from build123d import *

# Parameters (mm, degrees)
F0_W     = 500
F0_H     = 300
F1_DEPTH = 31.75
F2_R     = 1.5
F3_DEPTH = 31.751
F5_DEPTH = 12
F8_DEPTH = 31.751
F9_DEPTH = 19.05


# Not quite as in the source:
# - a length typed as a fraction of an inch, garbled in the dataset ("3 / 203.2 mm" for 3/8 in), is restored


with BuildPart() as f1:
    # F0 (on Top) → F1 (new body)
    with BuildSketch(Plane.XY):
        Rectangle(F0_W, F0_H)
    extrude(amount=-F1_DEPTH)

    # F2 (on Top) → F3 (cut, through all)
    with BuildSketch(Plane.XY):
        with Locations((-214.6335691214, 119.7834908962)):
            Circle(F2_R)
        with Locations((-214.6335691214, -117.7065091038)):
            Circle(F2_R)
        with Locations((207.7684308786, 119.7834908962)):
            Circle(F2_R)
        with Locations((207.7684308786, -117.7065091038)):
            Circle(F2_R)
        with Locations((630.1704308786, 119.7834908962)):
            Circle(F2_R)
        with Locations((630.1704308786, -117.7065091038)):
            Circle(F2_R)
    extrude(amount=-F3_DEPTH, mode=Mode.SUBTRACT)

    # F4 (on Top) → F5 (cut)
    with BuildSketch(Plane.XY):
        with BuildLine():
            ThreePointArc((-193.759300375, -80.4257169581), (-188.1796845566, -93.8961011397), (-174.709300375, -99.4757169581))
            Line((-174.709300375, -99.4757169581), (161.840699625, -99.4757169581))
            ThreePointArc((161.840699625, -99.4757169581), (175.3110838066, -93.8961011397), (180.890699625, -80.4257169581))
            Line((180.890699625, -80.4257169581), (180.890699625, 62.4492830419))
            ThreePointArc((180.890699625, 62.4492830419), (175.3110838066, 75.9196672235), (161.840699625, 81.4992830419))
            Line((161.840699625, 81.4992830419), (-174.709300375, 81.4992830419))
            ThreePointArc((-174.709300375, 81.4992830419), (-188.1796845566, 75.9196672235), (-193.759300375, 62.4492830419))
            Line((-193.759300375, 62.4492830419), (-193.759300375, -80.4257169581))
        make_face()
        with BuildLine():
            Line((210.890699625, 104.8424765468), (190.890699625, 104.8424765468))
            Line((190.890699625, 104.8424765468), (190.890699625, 11.4992830419))
            ThreePointArc((190.890699625, 11.4992830419), (200.890699625, 1.4992830419), (210.890699625, 11.4992830419))
            Line((210.890699625, 11.4992830419), (210.890699625, 104.8424765468))
        make_face()
    extrude(amount=-F5_DEPTH, mode=Mode.SUBTRACT)

    # F7 (on face) → F8 (cut, through all)
    with BuildSketch(Plane.XY):
        with BuildLine():
            Line((-174.709300375, -93.1257169581), (140.1676505526, -93.1257169581))
            Line((140.1676505526, -93.1257169581), (163.0281784434, -99.438670281))
            ThreePointArc((163.0281784434, -99.438670281), (175.7245746513, -93.4695091312), (180.890699625, -80.4257169581))
            Line((180.890699625, -80.4257169581), (180.890699625, 56.0992830419))
            Line((180.890699625, 56.0992830419), (154.220699625, 81.4992830419))
            Line((154.220699625, 81.4992830419), (-168.359300375, 81.4992830419))
            Line((-168.359300375, 81.4992830419), (-187.409300375, 62.4492830419))
            Line((-187.409300375, 62.4492830419), (-193.759300375, 56.0992830419))
            Line((-193.759300375, 56.0992830419), (-193.759300375, -74.0757169581))
            Line((-193.759300375, -74.0757169581), (-174.709300375, -93.1257169581))
        make_face()
    extrude(amount=-F8_DEPTH, mode=Mode.SUBTRACT)

    # F6 (on Top) → F9 (cut)
    with BuildSketch(Plane.XY):
        with BuildLine():
            ThreePointArc((-161.120300375, 111.4992830419), (-166.7055905698, 109.0628082362), (-168.7191172889, 103.3114965432))
            Line((-168.7191172889, 103.3114965432), (-167.089300375, 81.4992830419))
            Line((-167.089300375, 81.4992830419), (-93.429300375, 81.4992830419))
            Line((-93.429300375, 81.4992830419), (-91.799483461, 103.3114965432))
            ThreePointArc((-91.799483461, 103.3114965432), (-93.8130101802, 109.0628082362), (-99.398300375, 111.4992830419))
            Line((-99.398300375, 111.4992830419), (-161.120300375, 111.4992830419))
        make_face()
        with BuildLine():
            Line((148.251699625, 111.4992830419), (86.529699625, 111.4992830419))
            ThreePointArc((86.529699625, 111.4992830419), (80.9444094302, 109.0628082362), (78.9308827111, 103.3114965432))
            Line((78.9308827111, 103.3114965432), (80.560699625, 81.4992830419))
            Line((80.560699625, 81.4992830419), (154.220699625, 81.4992830419))
            Line((154.220699625, 81.4992830419), (155.850516539, 103.3114965432))
            ThreePointArc((155.850516539, 103.3114965432), (153.8369898198, 109.0628082362), (148.251699625, 111.4992830419))
        make_face()
    extrude(amount=-F9_DEPTH, mode=Mode.SUBTRACT)


solid = f1.part
Geometry: final body of the model. Coordinates: model frame, mm. A direction names the side the tool comes from. Give positions to 0.01 mm unless a question says otherwise; leave off trailing zeros. Write each loop counter-clockwise with the first axis right and the second up, starting at its lowest first coordinate (ties: lowest second). Pieces come first, ordered by that corner, then holes. Notation, with made-up numbers: (87, -14) - (138, -14) arc R34 ccw to (138, 21) - close; hole circle Ø11 at (11.5, 53). An arc over 180 degrees is marked (long way). Return JSON: item names as keys, results as strings. Group by question number.
1) Section C-C on z = -26. Return the cut outline in (x, y).
2) Set-up query: faces 4 (the flat face through (-3, 102, -31.75)), 5 (the flat face through (151.44, -96.24, -21.74)), 6 (the flat face through (210.891, 58, -6)). Return all of +Z, -Z, +X, -X, +Y, -Y with unobstructed straight access to the full face (end or side cutting, diameter ignored); none if empty.
3) Section B-B on y = -10.5. Return the cut outline in (x, z).
4) Section D-D on x = -21.5. Return the cut outline in (y, z).
5) First-contact query: P1, Ø2.5, axis at x = 207.77, y = 119.78, coming from the -Z side (3 decimals); P2, Ø20.5, axis at x = -98.5, y = -87, coming from the +Z side. Flat tips, straight axial feed; report the tip coordinate or a pass-through.
6) Section A-A on x = 103.5. Return the cut outline in (y, z), plus the area to 3 significant figures.
7) Line query: line 1 (X direction, y = 32, z = -10); line 2 (X direction, y = -60, z = -16); line 3 (Y direction, x = 104, z = -7). Output: solid intervals per line, ascending.
8) Mould query, pull axis X, two halves, no side actions, for faces 1 (the flat face through (-3, 150, -16)), 2 (the flat face through (-250, -2, -16)), 3 (the cylindrical face through (-188.327, -93.747, -5.916)). Classes: released by +X, released by -X, zero draft, split by the parting line, or undercut.
Filled in:
{
 "1": {"outline": "(-250, -150) - (250, -150) - (250, 150) - (-250, 150) - close; hole circle Ø3 at (-214.63, -117.71); hole circle Ø3 at (-214.63, 119.78); hole (-193.76, -74.08) - (-174.71, -93.13) - (140.17, -93.13) - (163.03, -99.44) arc R19.05 ccw to (180.89, -80.43) - (180.89, 56.1) - (154.22, 81.5) - (-168.36, 81.5) - (-193.76, 56.1) - close; hole circle Ø3 at (207.77, -117.71); hole circle Ø3 at (207.77, 119.78)"},
 "2": {"face 4": "-Z, +X, -X, +Y, -Y", "face 5": "+Z, -Z", "face 6": "+Z"},
 "3": {"outline": "(-250, -31.75) - (-193.76, -31.75) - (-193.76, 0) - (-250, 0) - close; (180.89, -31.75) - (250, -31.75) - (250, 0) - (180.89, 0) - close"},
 "4": {"outline": "(-150, -31.75) - (-93.13, -31.75) - (-93.13, -12) - (-99.48, -12) - (-99.48, 0) - (-150, 0) - close; (81.5, -31.75) - (150, -31.75) - (150, 0) - (81.5, 0) - close"},
 "5": {"P1": "passes through", "P2": "stops at z = -12"},
 "6": {"outline": "(-150, -31.75) - (-93.13, -31.75) - (-93.13, -12) - (-99.48, -12) - (-99.48, 0) - (-150, 0) - close; (81.5, -31.75) - (150, -31.75) - (150, 0) - (111.5, 0) - (111.5, -19.05) - (81.5, -19.05) - close", "area": "3,330 mm^2"},
 "7": {"line 1": "x = -250 to -193.76, 180.89 to 190.89, 210.89 to 250", "line 2": "x = -250 to -193.76, 180.89 to 250", "line 3": "y = -150 to -99.48, 111.5 to 150"},
 "8": {"face 1": "zero draft", "face 2": "released by -X", "face 3": "undercut"}
}
